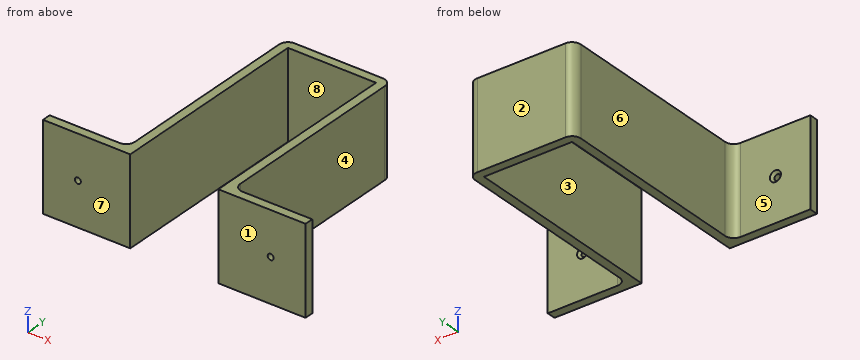
```python
from build123d import *

# Parameters (mm, degrees)
BOSS_EXTRU_1_DEPTH                             = 50
CONG_1_R                                       = 5
FRAISAGE_POUR_VIS_T_TE_FRAIS_E_M31_D           = 3.4
FRAISAGE_POUR_VIS_T_TE_FRAIS_E_M31_CSINK_D     = 6.3
FRAISAGE_POUR_VIS_T_TE_FRAIS_E_M31_CSINK_ANGLE = 90


with BuildPart() as part:
    # Esquisse1 → Boss.-Extru.1 (new body)
    with BuildSketch(Plane.XY):
        Polygon((-25.25, 0), (25.25, 0), (25.25, -118), (75.25, -118), (75.25, -113), (30.25, -113), (30.25, 5), (-30.25, 5), (-30.25, -113), (-75.25, -113), (-75.25, -118), (-25.25, -118), align=None)
    extrude(amount=BOSS_EXTRU_1_DEPTH)

    # Congé1
    cong_1_edges = [part.edges().sort_by_distance(p)[0] for p in [
        (-30.25, -113, 25),
        (-30.25, 5, 25),
        (30.25, 5, 25),
        (30.25, -113, 25),
    ]]
    fillet(cong_1_edges, radius=CONG_1_R)

    # Fraisage pour vis à tête fraisée M31 (through all)
    with Locations(Plane(origin=(0, -113, 0), x_dir=(1, 0, 0), z_dir=(0, 1, 0))):
        with Locations((-55.25, -25), (55.25, -25)):
            CounterSinkHole(FRAISAGE_POUR_VIS_T_TE_FRAIS_E_M31_D / 2, FRAISAGE_POUR_VIS_T_TE_FRAIS_E_M31_CSINK_D / 2, counter_sink_angle=FRAISAGE_POUR_VIS_T_TE_FRAIS_E_M31_CSINK_ANGLE)


solid = part.part
```
For this review, take the finished solid that the model builds, in its own axes (mm). Face numbers are marked on the shaded views. A direction names the side the tool comes from. Give positions to 0.01 mm unless a question says otherwise; leave off trailing zeros. Loops run counter-clockwise (first coordinate to the right, second up) from the corner with the lowest first, then second, coordinate; pieces in that order, holes last. Notation, with made-up numbers: M 64.25,49 L 83.25,49 A27 ccw 83.25,67 Z; hole C 35.5,52.5 d5. An arc over 180 degrees is marked long. One line per item, written item: value. Start each with the question number.
Q1. Draft analysis for pull direction X (two halves, no side actions). For the marked faces 6, 7 and 8, state which applies: released by +X, released by -X, zero draft, split by the parting line, or undercut.
Q2. Add section C-C (z = 25). Give the boundary of the cut face in (x, y).
Q3. Machinability: for the marked faces 1, 2, 3, 4 and 5, which of the approach directions +Z, -Z, +X, -X, +Y, -Y give a long, thin tool a straight path to every point of the face, cutting with its end or side? Answer none if there is none.
Q4. Add section B-B (x = 55.25). Give the boundary of the cut face in (y, z).
Q5. Clearance check with flat-ended pins moving along their axes: pin 1 Ø1.5 at (x, z) = (32, 36) entering from +Y; pin 2 Ø3 at (y, z) = (-67.5, 10) entering from +X; pin 3 Ø12 at (x, z) = (52, 19.5) entering from +Y. State where each tip first meets the part, or that it passes through.
Q6. Add section A-A (y = -4). Give the boundary of the cut face in (x, z).
Q7. For L1, parallel to X at y = -116, z = 25; L2, parallel to X at y = -47, z = 32; L3, parallel to Z at x = -55, y = -116, list the stretches that pass through material, from the lowest coordinate up.
Q8. Add section D-D (z = 6.5). Give the boundary of the cut face in (x, y).
Reply:
1. face 6: released by -X
1. face 7: zero draft
1. face 8: undercut
2. outline: M -75.25,-118 L -56.95,-118 L -56.95,-114.45 L -58.4,-113 L -75.25,-113 Z; M -53.55,-118 L -25.25,-118 L -25.25,0 L 25.25,0 L 25.25,-118 L 53.55,-118 L 53.55,-114.45 L 52.1,-113 L 35.25,-113 A5 cw 30.25,-108 L 30.25,0 A5 ccw 25.25,5 L -25.25,5 A5 ccw -30.25,0 L -30.25,-108 A5 cw -35.25,-113 L -52.1,-113 L -53.55,-114.45 Z; M 56.95,-118 L 75.25,-118 L 75.25,-113 L 58.4,-113 L 56.95,-114.45 Z
3. face 1: +Z, -Z, +X, -X, -Y
3. face 2: +Z, -Z, +X, -X, +Y
3. face 3: +Z, -Z, -Y
3. face 4: +Z, -Z, +X, +Y
3. face 5: +Z, -Z, -X, +Y
4. outline: M -118,0 L -113,0 L -113,21.85 L -114.45,23.3 L -118,23.3 Z; M -118,26.7 L -114.45,26.7 L -113,28.15 L -113,50 L -118,50 Z
5. pin 1: y = -111
5. pin 2: x = 30.25
5. pin 3: y = -113
6. outline: M -30.25,0 L -25.25,0 L -25.25,50 L -30.25,50 Z; M 25.25,0 L 30.25,0 L 30.25,50 L 25.25,50 Z
7. L1: -75.25 to -56.95, -53.55 to -25.25, 25.25 to 53.55, 56.95 to 75.25
7. L2: -30.25 to -25.25, 25.25 to 30.25
7. L3: 0 to 23.32, 26.68 to 50
8. outline: M -75.25,-118 L -25.25,-118 L -25.25,0 L 25.25,0 L 25.25,-118 L 75.25,-118 L 75.25,-113 L 35.25,-113 A5 cw 30.25,-108 L 30.25,0 A5 ccw 25.25,5 L -25.25,5 A5 ccw -30.25,0 L -30.25,-108 A5 cw -35.25,-113 L -75.25,-113 Z
